Could you check a few things on this drawing? It's one solid part, dimensions in mm from its lowest x, y, z. A direction names the side the tool comes from. Give positions to 0.01 mm unless a question says otherwise; leave off trailing zeros. Order: outer loops, then holes, each group sorted by start corner. A loop starts at its lowest first (then second) coordinate and runs counter-clockwise, first axis right, second up.
(1) Will these pins go through, and if not, where does the flat tip stop? pin 1 (2 mm diameter, centred on x = 21.5, z = 2.5, fed in from +Y); pin 2 (2.5 mm diameter, centred on x = 15.5, z = 13.5, fed in from -Y); pin 3 (2 mm diameter, centred on y = 6.5, z = 14.5, fed in from +X).
(2) Imagine slicing it at A-A, the plane y = 22.5. Write out the boundary of the cut face in (x, z) (1 decimal).
(3) On a 3-axis mill with a long thin cutter (end or side, diameter ignored), from which of +Z, -Z, +X, -X, +Y, -Y can I reach the whole of each face in a straight line? I mean the marked faces 1, 2 and 3. Say none if no direction works.
(4) Imagine slicing it at D-D, the plane y = 13.5. Write out the boundary of the cut face in (x, z), then the cut area to 3 significant figures.
(5) If we mould it in two halves opening along Y, with no side actions, what happens to the marked faces 4, 5 and 6? For each: released by +Y, released by -Y, zero draft, split by the parting line, or undercut.
(6) If I drill on probe 1 along Z at (x, y) = (20, 22.5) (1 decimal); probe 2 along Z at (x, y) = (8, 8); probe 3 along Y at (x, z) = (22.5, 1.75), over which ranges is the centre line in solid material (lowest first)?
(7) Imagine slicing it at B-B, the plane x = 32.5. Write out the boundary of the cut face in (y, z) (1 decimal).
(8) Imagine slicing it at C-C, the plane z = 13.5. Write out the boundary of the cut face in (x, y).
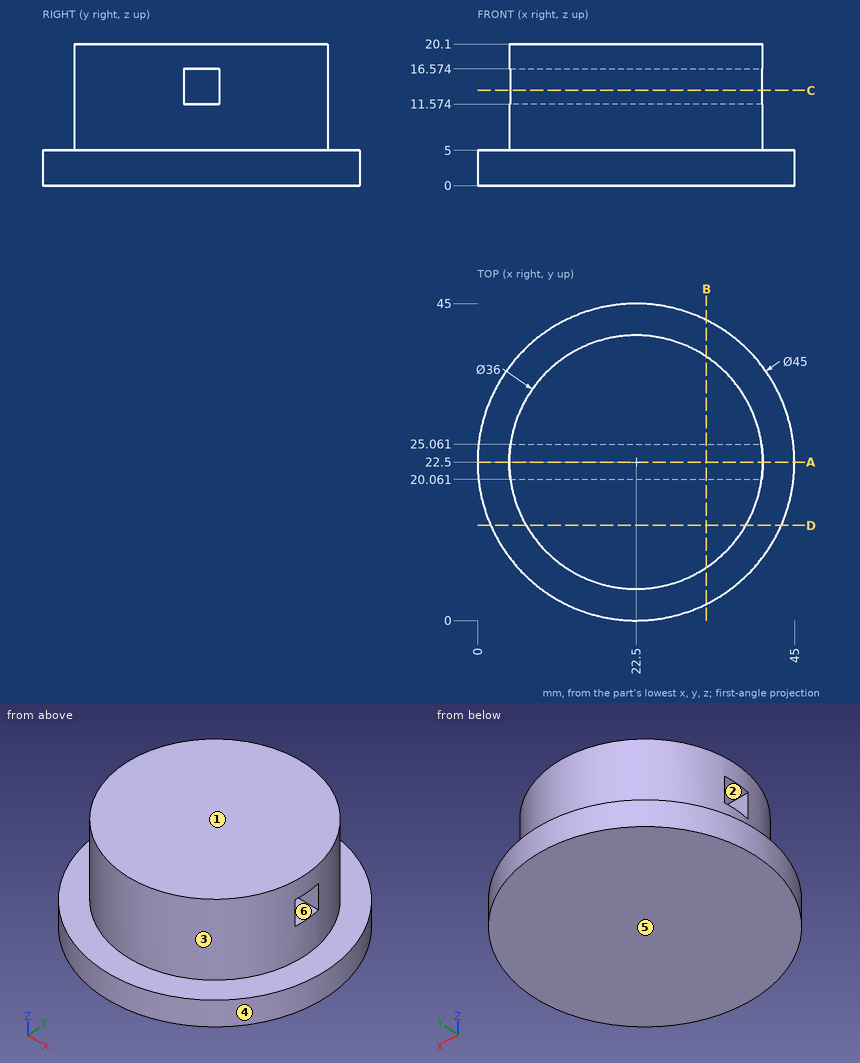
Answer block:
1. pin 1: stops at y = 45
1. pin 2: stops at y = 5.44
1. pin 3: stops at x = 32.45
2. outline: (0, 0) - (45, 0) - (45, 5) - (40.5, 5) - (40.5, 11.6) - (4.5, 11.6) - (4.5, 5) - (0, 5) - close; (4.5, 16.6) - (40.5, 16.6) - (40.5, 20.1) - (4.5, 20.1) - close
3. face 1: +Z, +X, -X, +Y, -Y
3. face 2: +X, -X
3. face 3: +Z
4. outline: (1.88, 0) - (43.12, 0) - (43.12, 5) - (38.09, 5) - (38.09, 20.1) - (6.91, 20.1) - (6.91, 5) - (1.88, 5) - close
4. area: 677 mm2
5. face 4: split by the parting line
5. face 5: zero draft
5. face 6: undercut
6. probe 1: z = 0 to 11.6, 16.6 to 20.1
6. probe 2: z = 0 to 5
6. probe 3: y = 0 to 45
7. outline: (2.3, 0) - (42.7, 0) - (42.7, 5) - (37.5, 5) - (37.5, 20.1) - (7.5, 20.1) - (7.5, 5) - (2.3, 5) - close; hole (20.1, 11.6) - (25.1, 11.6) - (25.1, 16.6) - (20.1, 16.6) - close
8. outline: (4.67, 20.06) arc R18 ccw to (40.33, 20.06) - close; (4.68, 25.06) - (40.32, 25.06) arc R18 ccw to start
